```python
from build123d import *

# Parameters (mm, degrees)
F2_R     = 4.7625
F3_DEPTH = 9.525
F5_R     = 12.7
F4_R     = 1.5875
F6_DEPTH = 14.3002


with BuildPart() as f1:
    # F0 (on Front) → F1 (revolve)
    with BuildSketch(Plane.XZ):
        Polygon((10.16, 55.764545), (10.16, 63.5), (0, 63.5), (0, 0), (31.75, 16.686577), (31.75, 28.86522), (31.75, 46.204952), (31.75, 55.764545), align=None)
    revolve(axis=Axis((0, 0, 31.75), (0, 0, -1)))

    # F2 (on face) → F3 (cut)
    with BuildSketch(Plane.XY.offset(63.5)):
        Circle(F2_R)
    extrude(amount=-F3_DEPTH, mode=Mode.SUBTRACT)

    # F5
    f5_edges = [f1.edges().sort_by_distance(p)[0] for p in [
        (-31.75, 0, 16.686577),
    ]]
    fillet(f5_edges, radius=F5_R)

    # F4 (on Top) → F6 (cut)
    with BuildSketch(Plane.XY):
        Circle(F4_R)
    extrude(amount=F6_DEPTH, mode=Mode.SUBTRACT)


solid = f1.part
```
Could you check a few things on this model? Use its own coordinates, in mm. A direction names the side the tool comes from. Coordinates: 2 decimals unless noted, no trailing zeros. Write each loop counter-clockwise with the first axis right and the second up, starting at its lowest first coordinate (ties: lowest second). Pieces come first, ordered by that corner, then holes. Notation, with made-up numbers: (-28, 36.5) -> (25, 36.5) arc R31 cw to (25, 67.5) -> close; hole circle Ø3 at (-29.75, -7). An arc over 180 degrees is marked (long way). One line per question, with ' | ' between items. Start each with the question number.
1. Please list where these lines run through material, in increasing order: line 1 along Y through (x, z) = (0, 57.5); line 2 along Y through (x, z) = (1, 55); line 3 along X through (y, z) = (1, 48).
2. Thinking about a two-plate mould opening in X: for faces 4 (the face through (-1.323, -10.074, 59.686)), 5 (the face through (-8, -8, 55.765)), 6 (the face through (-0.34, -1.55, 7.47)), which applies, pulls with the +X half, pulls with the -X half, needs draft (parallel to the pull), parting line crosses it, or undercut?
3. If we section it at A-A (z = 36.5): Please give me the cut outline in (x, y), and give its area (3 significant figures).
4. Will these pins go through, and if not, where does the flat tip stop? P1, Ø4, axis at x = -21, y = 17.5, coming from the +Z side; P2, Ø2.5, axis at x = 0, y = 0, coming from the +Z side (3 decimals); P3, Ø3, axis at x = -15.5, z = 29, coming from the +Y side.
5. For faces 1 (the face through (30.284, -9.537, 40.282)), 2 (the face through (-3.78, -2.9, 58.8)), 3 (the face through (0, 0, 14.3)), which set-ups out of +Z, -Z, +X, -X, +Y, -Y let a thin tool reach every point of the face, with its end or its side?
6. If we section it at B-B (z = 12): Please give me the cut outline in (x, y) (1 decimal), and give its area (3 significant figures).
Return value:
1) line 1: y = -10.16 to -4.76, 4.76 to 10.16 | line 2: y = -31.73 to -4.66, 4.66 to 31.73 | line 3: x = -31.73 to 31.73
2) face 4: parting line crosses it | face 5: needs draft | face 6: undercut
3) outline: circle Ø63.5 at (0, 0) | area: 3,170 mm²
4) P1: stops at z = 55.76 | P2: stops at z = 53.975 | P3: stops at y = 28.5
5) face 1: +Z, -Z | face 2: +Z | face 3: -Z
6) outline: circle Ø45.7 at (0, 0); hole circle Ø3.2 at (0, 0) | area: 1,630 mm²
